Build history of the part. All positions in model axes, mm. Give positions to 0.01 mm unless a question says otherwise; leave off trailing zeros. Order: outer loops, then holes, each group sorted by start corner. A loop starts at its lowest first (then second) coordinate and runs counter-clockwise, first axis right, second up. Notation, with made-up numbers: M 69,-16.75 L 76,-16.75 A28 cw 76,22.25 Z; hole C 33,17 d1. An arc over 180 degrees is marked long. One line per item, written item: value.
Autodesk Inventor part; units mm, degrees
ref_plane "Work Plane1" through (11.1612, 0, 0) normal (0, 0.866, -0.5) x (-1, 0, 0)
ref_plane "YZ Plane" through (0, 0, 0) normal (1, 0, 0) x (0, 1, 0)
ref_plane "XZ Plane" through (0, 0, 0) normal (0, 1, 0) x (-1, 0, 0)
sketch "Sketch1" plane through (0, 0, 0) normal (1, 0, 0) x (0, 1, 0)
  line L0 (4.0415, 0) -> (2.0207, -3.5)
  line L1 (2.0207, -3.5) -> (-2.0207, -3.5)
  line L2 (-2.0207, -3.5) -> (-4.0415, 0)
  line L3 (-4.0415, 0) -> (-2.0207, 3.5)
  line L4 (-2.0207, 3.5) -> (2.0207, 3.5)
  line L5 (2.0207, 3.5) -> (4.0415, 0)
  point P0 (0, 0)
  point P1 (0, 0)
  dimension "d0" = 8.0829
extrude "Body" add sketch "Sketch1" along normal blind 3.2
sketch "Sketch2" plane through (0, 0, 0) normal (-1, 0, 0) x (0, 0, 1)
  point P0 (0, 0)
hole "Thread" at (0, 0, 0) direction (1, 0, 0) diameter 3.242 end through all
chamfer "Chamfer1" distance 0.3789 angle 30 1 edges at (0, 0, -1.621) measured on face at (0, 2.4654, 1.4736)
chamfer "Chamfer2" distance 0.3789 angle 30 1 edges at (3.2, 0, -1.621) measured on face at (3.2, 2.4654, 1.4736)
sketch "Sketch3" plane through (0, 0, 0) normal (0, 0, 1) x (1, 0, 0)
  line L0 (0, 4.0415) -> (3.2, 4.0415)
  line L1 (3.2, 2.0207) -> (3.2, 4.0415)
  line L2 (-0.64, 0) -> (3.84, 0)
  line L3 (2.8874, 4.0415) -> (3.2, 3.5)
  dimension "d3" = 7
  dimension "d4" = 30
revolve "Chamfer3" cut sketch "Sketch3" angle 360 about axis through (-10, 0, 0) along (1, 0, 0)
ref_plane "Work Plane1" through (11.1612, 0, 0) normal (0, 0.866, -0.5) x (-1, 0, 0)
equation "\"d0\" = 1.1547 * SW"
equation "\"d1\" = KOH"
equation "\"d13\" = -0.5 * GD1 + 0.5 * NND"
equation "\"d21\" = -0.5 * GD1 + 0.5 * NND"
equation "\"d15\" = -0.5 * GD1 + 0.5 * NND"
equation "\"d22\" = -0.5 * GD1 + 0.5 * NND"
equation "\"d3\" = SW01"
equation "\"d4\" = ANG2"
equation "\"ANG2\" = 30deg"
equation "\"NND\" = 4"
equation "\"KOH\" = 3.2"
equation "\"SW\" = 7"
equation "\"SW01\" = SW"
equation "\"GUL\" = 0.541266 * PTC"
equation "\"TOA\" = 30deg"
equation "\"PTC\" = 0.7"
equation "\"E0\" = 1.155 * SW"
equation "\"THREADDIA\" = 4"
equation "\"GAL\" = 0.541266 * PTC"
properties part number "JIS B 1181 - HN - class 1 - Finished - M4" material "Steel, Mild"
1) Mould opens along Y. For faces 1 (the face through (0, 2, 2)), 2 (the face through (1.619, 1.438, 0.748)), 3 (the face through (1.6, -3, -1.8)) say: released by +Y, released by -Y, zero draft, split by the parting line, or undercut.
Check values:
face 1: zero draft
face 2: undercut
face 3: released by -Y
2) Saw through at A-A, the plane x = 2.55. Write the cut outline in (y, z), then the cut area to 3 significant figures.
Check values:
outline: M -4.04,0 L -2.02,-3.5 L 2.02,-3.5 L 4.04,0 L 2.02,3.5 L -2.02,3.5 Z; hole C 0,0 d3.24
area: 34.2 mm^2
3) Drill centre lines: probe 1 along Z at (x, y) = (1.8, 0); probe 2 along Y at (x, z) = (1.8, -0.5); probe 3 along Y at (x, z) = (1.9, 1). Where is each one in solid material? Low to high. Write a range as from..to.
Check values:
probe 1: -3.5..-1.62, 1.62..3.5
probe 2: -3.75..-1.54, 1.54..3.75
probe 3: -3.46..-1.28, 1.28..3.46
4) Pin check, flat tip, straight feed: pin 1 (1 mm diameter, centred on x = 1.5, z = 2.5, fed in from -Y). Stop position of the tip, or through.
Check values:
pin 1: y = -2.89
